The model under review builds one solid part; all positions refer to its coordinate system, in mm. Face numbers are marked on the shaded views. A direction names the side the tool comes from. Coordinates: 2 decimals unless noted, no trailing zeros. Order: outer loops, then holes, each group sorted by start corner. A loop starts at its lowest first (then second) coordinate and runs counter-clockwise, first axis right, second up. Notation, with made-up numbers: (83, 86) -> (140, 86) arc R27 ccw to (140, 106) -> close; hole circle Ø1 at (62.25, 81.25). An arc over 180 degrees is marked (long way). Answer as CSV lines item,"result". Start each with the question number.
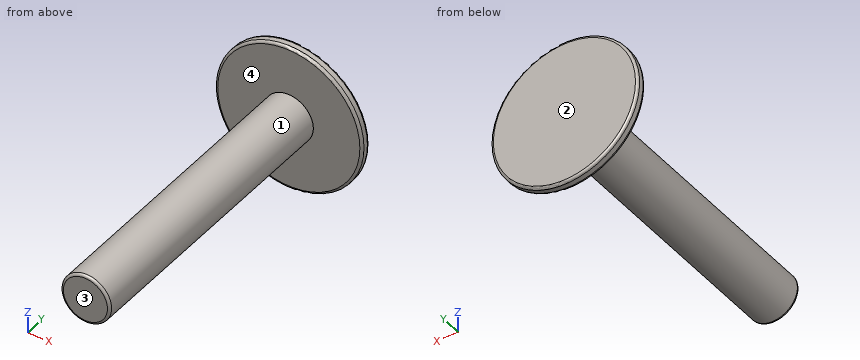
Autodesk Inventor part; units mm, degrees
ref_plane "YZ Plane" through (0, 0, 0) normal (1, 0, 0) x (0, 1, 0)
ref_plane "XZ Plane" through (0, 0, 0) normal (0, 1, 0) x (-1, 0, 0)
ref_plane "XY Plane" through (0, 0, 0) normal (0, 0, 1) x (1, 0, 0)
sketch "Boceto1" plane through (0, 0, 0) normal (0, 1, 0) x (-1, 0, 0)
  circle A0 centre (0, 0) radius 5
  dimension "d0" = 10
extrude "Extrusión1" add sketch "Boceto1" along normal blind 60
sketch "Boceto2" plane through (0, 60, 0) normal (0, 1, 0) x (1, 0, 0)
  circle A0 centre (0, 0) radius 15
  dimension "d3" = 30
extrude "Extrusión2" add sketch "Boceto2" along normal blind 2
fillet "Empalme1" radius 0.5 1 edges at (-15, 62, 0)
fillet "Empalme2" radius 0.5 1 edges at (-15, 60, 0)
fillet "Empalme3" radius 0.5 1 edges at (5, 0, 0)
properties part number "Pasador"
1) Mouldability with a two-part tool opening along X and no side actions: class the marked faces 1 and 2 as released by +X, released by -X, zero draft, split by the parting line, or undercut.
2) Consider section B-B (x = 0). Give the boundary of the cut face in (y, z), plus the area to 3 significant figures.
3) Tool access review of the marked faces 3 and 4: name each direction out of +Z, -Z, +X, -X, +Y, -Y from which nothing blocks a thin tool from reaching the whole face with its end or side.
4) Wall thickness on L1, parallel to Y at x = 8.5, z = 5.5; L2, parallel to Z at x = 0, y = 31; L3, parallel to X at y = 18, z = -2.5: over which ranges is each line inside the solid? List them lowest first. Write a range as [from, to].
5) Insertion check: pin 1 Ø1 at (y, z) = (49.5, 0) entering from -X; pin 2 Ø1 at (y, z) = (19.5, 1) entering from +X; pin 3 Ø12 at (x, y) = (-3, 47) entering from -Z. Each pin has a flat end and moves straight along its axis. Give the tip position at first contact, or say it passes through.
6) Consider section A-A (z = 0). Give the boundary of the cut face in (x, y), plus the area to 3 significant figures.
7) Consider section C-C (y = 20). Give the boundary of the cut face in (x, z), plus the area to 3 significant figures.
Result:
1,face 1,"split by the parting line"
1,face 2,"zero draft"
2,outline,"(0, -4.5) arc R0.5 ccw to (0.5, -5) -> (60, -5) -> (60, -14.5) arc R0.5 ccw to (60.5, -15) -> (61.5, -15) arc R0.5 ccw to (62, -14.5) -> (62, 14.5) arc R0.5 ccw to (61.5, 15) -> (60.5, 15) arc R0.5 ccw to (60, 14.5) -> (60, 5) -> (0.5, 5) arc R0.5 ccw to (0, 4.5) -> close"
2,area,"660 mm2"
3,face 3,"+Z, -Z, +X, -X, -Y"
3,face 4,"-Y"
4,L1,"[60, 62]"
4,L2,"[-5, 5]"
4,L3,"[-4.33, 4.33]"
5,pin 1,"x = -5"
5,pin 2,"x = 4.97"
5,pin 3,"z = -5"
6,outline,"(-15, 60.5) arc R0.5 ccw to (-14.5, 60) -> (-5, 60) -> (-5, 0.5) arc R0.5 ccw to (-4.5, 0) -> (4.5, 0) arc R0.5 ccw to (5, 0.5) -> (5, 60) -> (14.5, 60) arc R0.5 ccw to (15, 60.5) -> (15, 61.5) arc R0.5 ccw to (14.5, 62) -> (-14.5, 62) arc R0.5 ccw to (-15, 61.5) -> close"
6,area,"660 mm2"
7,outline,"circle Ø10 at (0, 0)"
7,area,"78.5 mm2"
